Source: CAD feature listing. Evaluate the final solid. Frame: model axes, mm. Face numbers are marked on the shaded views. A direction names the side the tool comes from. Round coordinates to 2 decimals unless told otherwise and drop trailing zeros. Write each loop counter-clockwise with the first axis right and the second up, starting at its lowest first coordinate (ties: lowest second). Pieces come first, ordered by that corner, then holes. Notation, with made-up numbers: (72.5, -27) - (84.5, -27) arc R28 cw to (84.5, -2) - close; hole circle Ø2 at (70.5, 78.5). An arc over 180 degrees is marked (long way). Write item = value, one per line. Start each with the question number.
```python
from build123d import *

# Parameters (mm, degrees)
BOSS_EXTRUDE1_DEPTH      = 70
SKETCH7_W                = 114
SKETCH7_H                = 64
CUT_EXTRUDE2_DEPTH       = 77
SKETCH8_W                = 3
SKETCH8_H                = 64
BOSS_EXTRUDE3_DEPTH      = 114
BOSS_EXTRUDE4_REACH      = 117.47
BOSS_EXTRUDE4_END_RADIUS = 150
SKETCH9_W                = 114
SKETCH9_H                = 3
SKETCH10_R               = 2
CUT_EXTRUDE3_DEPTH       = 3


with BuildPart() as part:
    # Sketch1 → Boss-Extrude1 (new body)
    with BuildSketch(Plane(origin=(0, 0, 0), x_dir=(1, 0, 0), z_dir=(0, 1, 0))):
        with BuildLine():
            Line((-60, 137.477270849), (-60, 77.477270849))
            Line((-60, 77.477270849), (60, 77.477270849))
            Line((60, 77.477270849), (60, 137.477270849))
            ThreePointArc((60, 137.477270849), (0, 150), (-60, 137.477270849))
        make_face()
    extrude(amount=BOSS_EXTRUDE1_DEPTH)

    # Sketch7 → Cut-Extrude2 (cut)
    with BuildSketch(Plane.XY.offset(-77.477270849)):
        with Locations((0, 35)):
            Rectangle(SKETCH7_W, SKETCH7_H)
    extrude(amount=-CUT_EXTRUDE2_DEPTH, mode=Mode.SUBTRACT)

    # Sketch8 → Boss-Extrude3 (add)
    with BuildSketch(Plane(origin=(-57, 0, 0), x_dir=(0, 0, -1), z_dir=(1, 0, 0))):
        with Locations((78.977270849, 35)):
            Rectangle(SKETCH8_W, SKETCH8_H)
    extrude(amount=BOSS_EXTRUDE3_DEPTH)

    # Boss-Extrude4: up to this cylinder (the profile starts inside it)
    boss_extrude4_end = Plane(origin=(0, 35, 0), z_dir=(0, -1, 0)) * Cylinder(BOSS_EXTRUDE4_END_RADIUS, 535.94, mode=Mode.PRIVATE)
    # Sketch9 → Boss-Extrude4 (add, up to the surface)
    with BuildSketch(Plane(origin=(0, 0, -80.477270849), x_dir=(-1, 0, 0), z_dir=(0, 0, -1)), mode=Mode.PRIVATE) as boss_extrude4_sk1:
        with Locations((0, 35)):
            Rectangle(SKETCH9_W, SKETCH9_H)
    boss_extrude4_tool1 = extrude(boss_extrude4_sk1.sketch, amount=BOSS_EXTRUDE4_REACH, mode=Mode.PRIVATE) & boss_extrude4_end
    add(boss_extrude4_tool1.solids().sort_by_distance((0, 35, -80.477271))[0])

    # Sketch10 → Cut-Extrude3 (cut)
    with BuildSketch(Plane(origin=(0, 70, 0), x_dir=(1, 0, 0), z_dir=(0, 1, 0))):
        with Locations(Location((-35, 104.997270849, 0), (0, 0, 270))):
            Circle(SKETCH10_R)
        with Locations(Location((35, 104.997270849, 0), (0, 0, 270))):
            Circle(SKETCH10_R)
    extrude(amount=-CUT_EXTRUDE3_DEPTH, mode=Mode.SUBTRACT)


solid = part.part
```
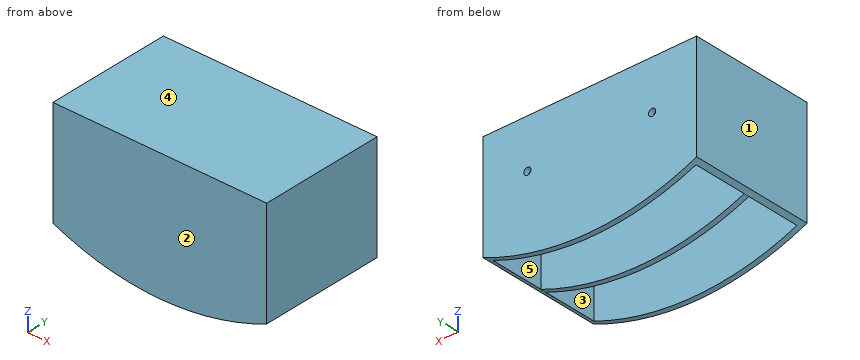
(1) Contact query for flat-ended pins moving along their axis: P1, Ø10, axis at x = -9, y = 35.5, coming from the -Z side; P2, Ø15, axis at x = 17, y = 23, coming from the -Z side; P3, Ø2.5, axis at x = 35, z = -105, coming from the +Y side. Output: stop coordinate, or through.
(2) Reachability of the marked faces 4 and 5 from +Z, -Z, +X, -X, +Y, -Y: full face, straight path, thin tool, end or side. Return the list, or none.
(3) Ray query, L1, parallel to Y at x = 41, z = -143.5; L2, parallel to X at y = 26.5, z = -81; L3, parallel to Z at x = 19, y = 63.5. Return the intervals inside material, ascending. Write a range as from..to.
(4) Pull-direction query (X, two-part tool) for the marked faces 1, 2 and 3; classes: +X half, -X half, draft (parallel to the pull), parting line (faces both ways), or undercut.
(5) Section B-B (z = -144.5). Return the cut outline in (x, y).
(6) Section D-D (y = 38.5). Return the cut outline in (x, z).
(7) Section A-A (z = -84.5). Return the cut outline in (x, y).
(8) Section C-C (x = -35). Return the cut outline in (y, z), plus the area to 3 significant figures.
Solution:
q1.P1 = -149.95
q1.P2 = -80.48
q1.P3 = 36.5
q2.face_4 = +Z, +X, -X, +Y, -Y
q2.face_5 = -Z
q3.L1 = 0..3, 33.5..36.5, 67..70
q3.L2 = -60..-57, 57..60
q3.L3 = -80.48..-77.48
q4.face_1 = -X half
q4.face_2 = draft
q4.face_3 = undercut
q5.outline = (-40.25, 0) - (40.25, 0) - (40.25, 3) - (-40.25, 3) - close; (-40.25, 33.5) - (40.25, 33.5) - (40.25, 36.5) - (-40.25, 36.5) - close; (-40.25, 67) - (40.25, 67) - (40.25, 70) - (-40.25, 70) - close
q6.outline = (-60, -137.48) arc R150 ccw to (-57, -138.75) - (-57, -80.48) - (57, -80.48) - (57, -138.75) arc R150 ccw to (60, -137.48) - (60, -77.48) - (-60, -77.48) - close
q7.outline = (-60, 0) - (60, 0) - (60, 70) - (-60, 70) - close; hole (-57, 3) - (57, 3) - (57, 33.5) - (-57, 33.5) - close; hole (-57, 36.5) - (57, 36.5) - (57, 67) - (-57, 67) - close
q8.outline = (0, -145.86) - (3, -145.86) - (3, -80.48) - (33.5, -80.48) - (33.5, -145.86) - (36.5, -145.86) - (36.5, -80.48) - (67, -80.48) - (67, -103) - (70, -103) - (70, -77.48) - (0, -77.48) - close; (67, -145.86) - (70, -145.86) - (70, -107) - (67, -107) - close
q8.area = 786 mm^2
